from build123d import *

# Parameters (mm, degrees)
F1_DEPTH = 63.5
F0_W     = 19.3484129535
F0_H     = 19.05
F0_H_2   = 4.7498
F0_H_3   = 4.7752
F2_DEPTH = 25.4
F3_DEPTH = 7.9375
F4_R     = 6.35


with BuildPart() as f1:
    # F0 (on Front) → F1 (new body, symmetric)
    with BuildSketch(Plane.XZ):
        Polygon((-41.275, 18.6743041574), (-41.275, -0.3756958426), (41.275, -0.3756958426), (41.275, 18.6743041574), (22.225, 18.6743041574), align=None)
    extrude(amount=F1_DEPTH, both=True)

    # F0 (on Front) → F2 (join, symmetric)
    with BuildSketch(Plane.XZ):
        with BuildLine():
            Line((22.225, 18.6743041574), (41.275, 18.6743041574))
            Line((41.275, 18.6743041574), (41.275, 36.1495041574))
            ThreePointArc((41.275, 36.1495041574), (45.9246798487, 47.3748243087), (57.15, 52.0245041574))
            Line((57.15, 52.0245041574), (60.325, 52.0245041574))
            Line((60.325, 52.0245041574), (60.325, 71.0745041574))
            Line((60.325, 71.0745041574), (57.15, 71.0745041574))
            ThreePointArc((57.15, 71.0745041574), (32.4542956671, 60.8452084903), (22.225, 36.1495041574))
            Line((22.225, 36.1495041574), (22.225, 18.6743041574))
        make_face()
        Polygon((79.6734129535, 75.8243041574), (79.6734129535, 71.0745041574), (79.6734129535, 52.0245041574), (79.6734129535, 47.2493041574), (111.125, 47.2493041574), (111.125, 75.8243041574), align=None)
        with Locations((69.9992064767, 61.5495041574)):
            Rectangle(F0_W, F0_H)
        with Locations((69.9992064767, 73.4494041574)):
            Rectangle(F0_W, F0_H_2)
        with Locations((69.9992064767, 49.6369041574)):
            Rectangle(F0_W, F0_H_3)
    extrude(amount=F2_DEPTH, both=True)

    # F0 (on Front) → F3 (join, symmetric)
    with BuildSketch(Plane.XZ):
        with BuildLine():
            add(Edge.make_bspline(
                [(-41.275, 18.6743041574), (-22.7171909064, 55.2262067795), (18.2569045573, 71.5698078275), (57.15, 71.0745041574)],
                knots=[0, 0, 0, 0, 111.5045361635, 111.5045361635, 111.5045361635, 111.5045361635], degree=3))
            Line((-41.275, 18.6743041574), (22.225, 18.6743041574))
            Line((22.225, 18.6743041574), (22.225, 36.1495041574))
            ThreePointArc((22.225, 36.1495041574), (32.4542956671, 60.8452084903), (57.15, 71.0745041574))
        make_face()
    extrude(amount=F3_DEPTH, both=True)

    # F4
    f4_edges = [f1.edges().sort_by_distance(p)[0] for p in [
        (-41.275, 63.5, 9.149304),
        (-41.275, -63.5, 9.149304),
        (41.275, 63.5, 9.149304),
        (41.275, -63.5, 9.149304),
    ]]
    fillet(f4_edges, radius=F4_R)


solid = f1.part
Check sheet for the modelled part. Datum: model origin and axes. Units: mm. A direction names the side the tool comes from. Give positions to 0.01 mm unless a question says otherwise; leave off trailing zeros. Write each loop counter-clockwise with the first axis right and the second up, starting at its lowest first coordinate (ties: lowest second). Pieces come first, ordered by that corner, then holes. Notation, with made-up numbers: M 61.25,55.25 L 85.25,55.25 A33 cw 85.25,88.25 Z; hole C 45.25,75 d7. An arc over 180 degrees is marked long. Use one line per item in the form item = value.
(1) Draft check along X on faces 4 (the cylindrical face through (39.365, 61.689, 9.283)), 5 (the cylindrical face through (45.8, -0.36, 47.25)), 6 (the flat face through (-41.275, -1, 9)). Enter one of: pulls with the +X half, pulls with the -X half, needs draft (parallel to the pull), parting line crosses it, or undercut.
Answer block:
face_4 = pulls with the +X half
face_5 = undercut
face_6 = pulls with the -X half
(2) Section check B-B on z = 5. Record the boundary of the cut face in (x, y) (3 decimals).
Answer block:
outline = M -41.275,-57.15 A6.35 ccw -34.925,-63.5 L 34.925,-63.5 A6.35 ccw 41.275,-57.15 L 41.275,57.15 A6.35 ccw 34.925,63.5 L -34.925,63.5 A6.35 ccw -41.275,57.15 Z
(3) Tool access check on faces 1 (the flat face through (-2, 7.938, 40)), 2 (the flat face through (66, -25.4, 54)), 3 (the cylindrical face through (32.73, -16.79, 61.12)). Record the directions out of +Z, -Z, +X, -X, +Y, -Y that give a thin tool (end or side, any length) a straight path to the whole face; none if there is none.
Answer block:
face_1 = +Z, -X, +Y
face_2 = +Z, +X, -X, -Y
face_3 = +Z, -X, -Y
(4) Section check C-C on x = 68. Record the boundary of the cut face in (y, z), plus the area to 3 significant figures.
Answer block:
outline = M -25.4,47.25 L 25.4,47.25 L 25.4,75.82 L -25.4,75.82 Z
area = 1,450 mm2
(5) Depth check by flat-ended pin: P1, Ø17, axis at x = 48, z = 55, coming from the +Y side; P2, Ø11, axis at y = 18.5, z = 26, coming from the +X side (3 decimals); P3, Ø8.5, axis at y = 14, z = 23.5, coming from the -X side (3 decimals). Enter the tip coordinate at first touch or a pass-through.
Answer block:
P1 = 25.4
P2 = 41.275
P3 = 22.225
(6) Material ranges on line 1 along Z through (x, y) = (-31, -33.5); line 2 along Y through (x, z) = (20, 38.5); line 3 along X through (y, z) = (-8, 20) (3 decimals), recorded low to high.
Answer block:
line_1 = -0.38 to 18.67
line_2 = -7.94 to 7.94
line_3 = 22.225 to 41.275
